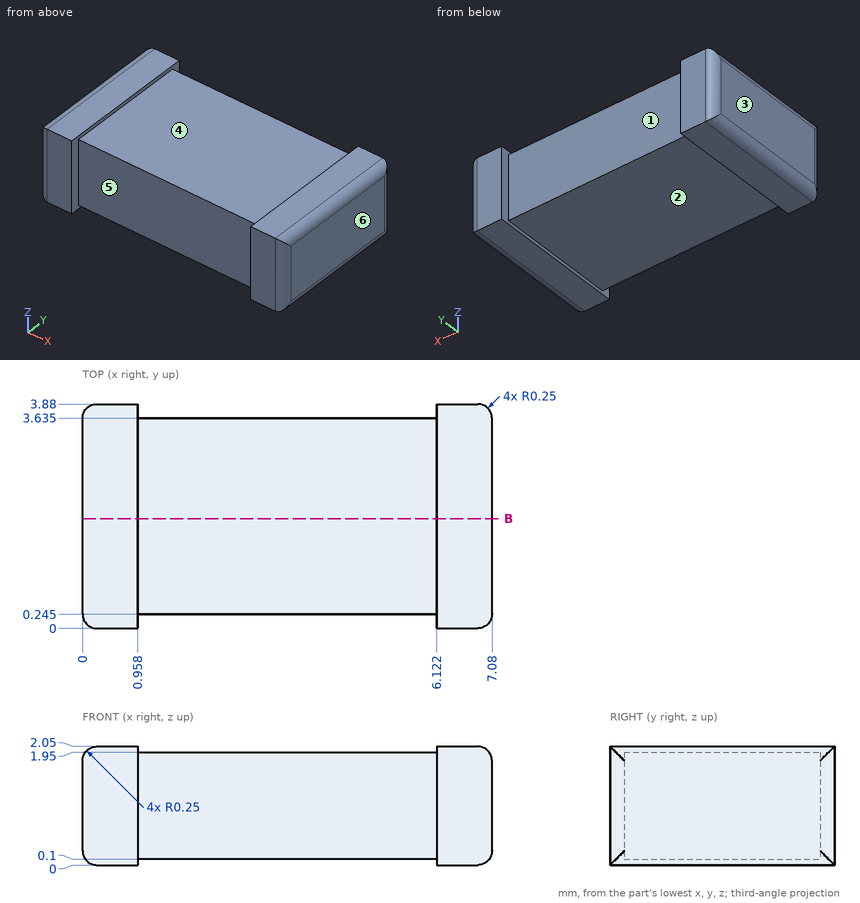
Check sheet for the drawn part. Datum: minimum x, y, z corner. Units: mm. A direction names the side the tool comes from. Give positions to 0.01 mm unless a question says otherwise; leave off trailing zeros. Write each loop counter-clockwise with the first axis right and the second up, starting at its lowest first coordinate (ties: lowest second). Pieces come first, ordered by that corner, then holes. Notation, with made-up numbers: (7.5, 8.25) - (14.5, 8.25) arc R27 cw to (14.5, 39.25) - close; hole circle Ø9 at (72.5, 11.25). An arc over 180 degrees is marked (long way). Put each result on its own line as item: value.
1. Thickness scan on line 1 (Z direction, x = 2, y = 3.3); line 2 (Y direction, x = 2.5, z = 1.25) (1 decimal); line 3 (X direction, y = 1.2, z = 0.15). Record the ranges inside material, lowest first.
Ans:
line 1: z = 0.1 to 1.95
line 2: y = 0.2 to 3.6
line 3: x = 0.02 to 7.06
2. Go/stop test with flat-tipped pins: pin 1 (1.5 mm diameter, centred on x = 1, y = 3, fed in from -Z); pin 2 (0.6 mm diameter, centred on x = 4, z = 1, fed in from +Y) (1 decimal); pin 3 (1.7 mm diameter, centred on x = 4.5, y = 2.5, fed in from +Z); pin 4 (1 mm diameter, centred on x = 4.5, z = 1.5, fed in from -Y) (1 decimal). Record where each tip stops, or that it passes through.
Ans:
pin 1: stops at z = 0
pin 2: stops at y = 3.6
pin 3: stops at z = 1.95
pin 4: stops at y = 0.2
3. Sectioned sample at B-B, the plane y = 1.9. Enter the section's corners in (x, z), plus the area to 3 significant figures.
Ans:
outline: (0, 0.25) arc R0.25 ccw to (0.25, 0) - (0.96, 0) - (0.96, 0.1) - (6.12, 0.1) - (6.12, 0) - (6.83, 0) arc R0.25 ccw to (7.08, 0.25) - (7.08, 1.8) arc R0.25 ccw to (6.83, 2.05) - (6.12, 2.05) - (6.12, 1.95) - (0.96, 1.95) - (0.96, 2.05) - (0.25, 2.05) arc R0.25 ccw to (0, 1.8) - close
area: 13.4 mm²
4. Draft check along X on the marked faces 3, 4, 5 and 6. Enter one of: +X half, -X half, draft (parallel to the pull), parting line (faces both ways), or undercut.
Ans:
face 3: -X half
face 4: undercut
face 5: undercut
face 6: +X half
5. Set-up check for the marked faces 1 and 2: record each of +Z, -Z, +X, -X, +Y, -Y from which the full face is reachable in a straight line by a thin tool's end or side.
Ans:
face 1: +Z, -Z, +Y
face 2: -Z, +Y, -Y
